The model under review builds one solid part; all positions refer to its coordinate system, in mm. Round coordinates to 2 decimals unless told otherwise and drop trailing zeros. Order: outer loops, then holes, each group sorted by start corner. A loop starts at its lowest first (then second) coordinate and runs counter-clockwise, first axis right, second up.
```python
from build123d import *

# Parameters (mm, degrees)
SKETCH1_W           = 90
SKETCH1_H           = 120
BOSS_EXTRUDE1_DEPTH = 8
SKETCH2_R           = 5
CUT_EXTRUDE1_DEPTH  = 9
SKETCH3_R           = 2
CUT_EXTRUDE2_DEPTH  = 9
SKETCH4_R           = 2
CUT_EXTRUDE3_DEPTH  = 9


with BuildPart() as part:
    # Sketch1 → Boss-Extrude1 (new body)
    with BuildSketch(Plane.XY):
        with Locations((45, 60)):
            Rectangle(SKETCH1_W, SKETCH1_H)
    extrude(amount=BOSS_EXTRUDE1_DEPTH)

    # Sketch2 → Cut-Extrude1 (cut, through all)
    with BuildSketch(Plane.XY.offset(8)):
        with Locations((70, 64)):
            Circle(SKETCH2_R)
    extrude(amount=-CUT_EXTRUDE1_DEPTH, mode=Mode.SUBTRACT)

    # Sketch3 → Cut-Extrude2 (cut, through all)
    with BuildSketch(Plane.XY.offset(8)):
        with Locations((87, 70)):
            Circle(SKETCH3_R)
        with Locations((60.5, 46.7)):
            Circle(SKETCH3_R)
    extrude(amount=-CUT_EXTRUDE2_DEPTH, mode=Mode.SUBTRACT)

    # Sketch4 → Cut-Extrude3 (cut, through all)
    with BuildSketch(Plane.XY.offset(8)):
        with Locations((50.5, 96.5)):
            Circle(SKETCH4_R)
        with Locations((10.5, 96.5)):
            Circle(SKETCH4_R)
        with Locations((50.5, 41.5)):
            Circle(SKETCH4_R)
        with Locations((10.5, 41.5)):
            Circle(SKETCH4_R)
    extrude(amount=-CUT_EXTRUDE3_DEPTH, mode=Mode.SUBTRACT)


solid = part.part
```
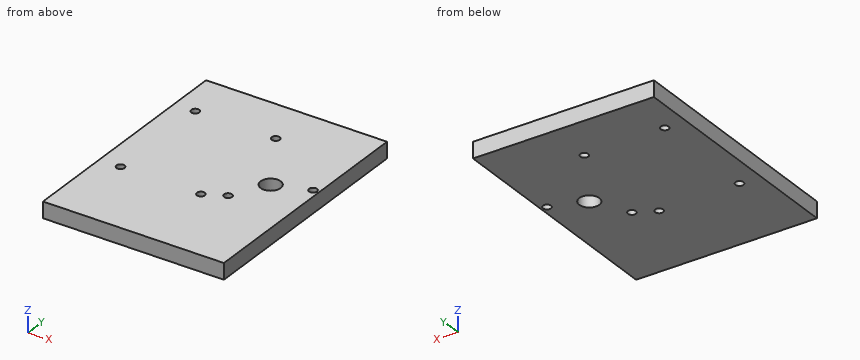
(1) Consider section C-C (x = 60.5). Write out the cut boundary in (y, z).
Data:
outline: (0, 0) - (44.7, 0) - (44.7, 8) - (0, 8) - close; (48.7, 0) - (120, 0) - (120, 8) - (48.7, 8) - close
(2) Consider section A-A (y = 46.7). Write out the cut boundary in (x, z).
Data:
outline: (0, 0) - (58.5, 0) - (58.5, 8) - (0, 8) - close; (62.5, 0) - (90, 0) - (90, 8) - (62.5, 8) - close
(3) To check wall thickness, follow probe 1 along Y at (x, z) = (10.5, 6); probe 2 along Y at (x, z) = (87, 3.5); probe 3 along Y at (x, z) = (70, 3). State the ranges of each line that lie inside material, in increasing order.
Data:
probe 1: y = 0 to 39.5, 43.5 to 94.5, 98.5 to 120
probe 2: y = 0 to 68, 72 to 120
probe 3: y = 0 to 59, 69 to 120
(4) Consider section B-B (x = 10.5). Write out the cut boundary in (y, z).
Data:
outline: (0, 0) - (39.5, 0) - (39.5, 8) - (0, 8) - close; (43.5, 0) - (94.5, 0) - (94.5, 8) - (43.5, 8) - close; (98.5, 0) - (120, 0) - (120, 8) - (98.5, 8) - close
